Model file for the job. Use its own axes, mm. A direction names the side the tool comes from. Round coordinates to 2 decimals unless told otherwise and drop trailing zeros. Order: outer loops, then holes, each group sorted by start corner. A loop starts at its lowest first (then second) coordinate and runs counter-clockwise, first axis right, second up. Notation, with made-up numbers: M 76.25,6 L 119.25,6 A16 cw 119.25,31 Z; hole C 50,-37.5 d7. An arc over 180 degrees is marked long. Return JSON: item names as keys, results as strings. Group by question number.
Item 1: Pin check, flat tips, straight feed: pin 1 Ø10 at (x, y) = (9.5, 7.5) entering from -Z; pin 2 Ø0.8 at (x, z) = (0, 0.5) entering from -Y; pin 3 Ø4.5 at (y, z) = (8, 3) entering from -X; pin 4 Ø2 at (y, z) = (-8, -1.5) entering from +X. Stop position of each tip, or through.
Item 2: Which spindle directions (+Z, -Z, +X, -X, +Y, -Y) get a long thin tool onto all of the face, cutting with end or side? Do faces 4 (the face through (-5.1, -0.1, 0.7)), 5 (the face through (-7.5, -6, 0)), 6 (the face through (0.75, 7, 1)), 7 (the face through (6.5, -0.1, 4.5)), 8 (the face through (-5.21, -0.1, -3.71)). Say none if no direction does.
Item 3: Slice it at A-A on y = 0. Write the cut outline in (x, z), then the cut area to 3 significant figures.
Item 4: Slice it at C-C on x = 0. Write the cut outline in (y, z).
Item 5: Pull direction X, two halves, no side cores. Call faces 1 (the face through (-0.75, -9, 2)), 2 (the face through (-5.7, 0.4, 5.5)), 3 (the face through (-6.14, -0.13, 5.36)): pulls with the +X half, pulls with the -X half, needs draft (parallel to the pull), parting line crosses it, or undercut.
Item 6: Slice it at B-B on z = 0. Write the cut outline in (x, y), then the cut area to 3 significant figures.
Item 7: Probe line 1 along X through (y, z) = (8, 2); line 2 along X through (y, z) = (0, -1.5); line 3 along Z through (x, y) = (-8.8, -8). List the from-to ranges inside material, lowest first.
Autodesk Inventor part; units mm, degrees
ref_plane "body_screw_XY" through (4, -8, 0) normal (1, 0, 0) x (0, 0, -1)
ref_plane "body_screw_YZ" through (4, -8, 0) normal (0, 0, -1) x (0, 1, 0)
ref_plane "body_screw_ZX" through (4, -8, 0) normal (0, 1, 0) x (1, 0, 0)
sketch "Sketch_1" plane through (0, 0, 0) normal (1, 0, 0) x (0, 1, 0)
  line L0 (0, -4) -> (0, 5.5)
  line L1 (6, 5.5) -> (5.5, 5.5)
  line L2 (5.5, 5.5) -> (5, 5)
  line L3 (5, 5) -> (5, -3.5)
  line L4 (5, -3.5) -> (5.5, -4)
  line L5 (5.5, -4) -> (12, -4)
  line L6 (12, -4) -> (12.5, -3.5)
  line L7 (12.5, -3.5) -> (12.5, 3.5)
  line L8 (12.5, 3.5) -> (12, 4)
  line L9 (12, 4) -> (6.5, 4)
  line L10 (6.5, 4) -> (6.5, 5)
  line L11 (6.5, 5) -> (6, 5.5)
revolve "Revolution1" add sketch "Sketch_1" angle 360 about axis through (0, 0, -4) along (0, 0, -1)
sketch "Sketch_2" plane through (0, 0, 0) normal (0, 0, 1) x (1, 0, 0)
  line L0 (-0.75, -12.5) -> (0.75, -12.5)
  line L1 (0.75, -12.5) -> (0.75, 9)
  line L2 (0.75, 9) -> (-0.75, 9)
  line L3 (-0.75, 9) -> (-0.75, -12.5)
extrude "Extrusion1" cut sketch "Sketch_2" along normal mid plane 32
sketch "Sketch_3" plane through (0, 0, 0) normal (0, 0, 1) x (1, 0, 0)
  line L0 (0, -8) -> (12.5, -8)
  line L1 (12.5, -8) -> (12.5, -11)
  line L2 (12.5, -11) -> (4, -11)
  line L3 (4, -11) -> (4, -9.75)
  line L4 (4, -9.75) -> (0, -9.75)
  line L5 (0, -9.75) -> (0, -8)
  line L6 (0, -8) -> (12.5, -8)
ref_plane "body_screw_XY" through (4, -8, 0) normal (1, 0, 0) x (0, 0, -1)
ref_plane "body_screw_YZ" through (4, -8, 0) normal (0, 0, -1) x (0, 1, 0)
ref_plane "body_screw_ZX" through (4, -8, 0) normal (0, 1, 0) x (1, 0, 0)
sketch "スケッチ5" plane through (0, 0, -4) normal (0, 0, -1) x (-1, 0, 0)
  circle A0 centre (0, 0) radius 5.1
  dimension "d12" = 10.2
extrude "押し出し2" cut sketch "スケッチ5" against normal through all
ref_plane "作業平面4" through (12.5, 0, 0) normal (1, 0, 0) x (0, 1, 0)
sketch "スケッチ6" plane through (12.5, 0, 0) normal (1, 0, 0) x (0, 1, 0)
  circle A0 centre (-8, 0) radius 1.75
  circle A1 centre (-8, 0) radius 1.7
  circle A2 centre (-8, 0) radius 3.5
  point P0 (0, 0)
  dimension "d15" = 3.4
  dimension "d16" = 7
extrude "押し出し3" cut sketch "スケッチ6" against normal through all contours A1
extrude "押し出し4" cut sketch "スケッチ6" against normal blind 8.5 contours A0 | A2
ref_plane "作業平面5" through (-12.5, 0, 0) normal (1, 0, 0) x (0, 1, 0)
extrude "押し出し5" cut sketch "スケッチ6" along normal blind 5 from surface at -25 contours A0 | A2
properties part number "PSCBNJ10-13b"
Output values:
{
 "1": {"pin 1": "z = -4", "pin 2": "y = 9", "pin 3": "x = -11.1", "pin 4": "x = 4"},
 "2": {"face 4": "+Z, -Z", "face 5": "-X", "face 6": "+Z, -Z, -Y", "face 7": "+Z, +X", "face 8": "-Z"},
 "3": {"outline": "M -12.5,-3.5 L -12,-4 L -5.5,-4 L -5.1,-3.6 L -5.1,5.1 L -5.5,5.5 L -6,5.5 L -6.5,5 L -6.5,4 L -12,4 L -12.5,3.5 Z; M 5.1,-3.6 L 5.5,-4 L 12,-4 L 12.5,-3.5 L 12.5,3.5 L 12,4 L 6.5,4 L 6.5,5 L 6,5.5 L 5.5,5.5 L 5.1,5.1 Z", "area": "122 mm²"},
 "4": {"outline": "M 9,-4 L 12,-4 L 12.5,-3.5 L 12.5,3.5 L 12,4 L 9,4 Z"},
 "5": {"face 1": "undercut", "face 2": "needs draft", "face 3": "pulls with the -X half"},
 "6": {"outline": "M -11.66,-4.5 L -7.5,-4.5 L -7.5,-6.3 L -0.75,-6.3 L -0.75,-5.04 A5.1 cw -0.75,5.04 L -0.75,9 L 0.75,9 L 0.75,5.04 A5.1 cw 0.75,-5.04 L 0.75,-6.3 L 4,-6.3 L 4,-4.5 L 11.66,-4.5 A12.5 ccw long Z; M -7.5,-10 A12.5 ccw -0.75,-12.48 L -0.75,-9.7 L -7.5,-9.7 Z; M 0.75,-12.48 A12.5 ccw 4.9,-11.5 L 4,-11.5 L 4,-9.7 L 0.75,-9.7 Z", "area": "308 mm²"},
 "7": {"line 1": "-9.6 to -0.75, 0.75 to 9.6", "line 2": "-12.5 to -5.1, 5.1 to 12.5", "line 3": "-4 to -3.5, 3.5 to 4"}
}
